Part model, mm, in its own coordinate system. Face numbers are marked on the shaded views. A direction names the side the tool comes from. Round coordinates to 2 decimals unless told otherwise and drop trailing zeros. Loops run counter-clockwise (first coordinate to the right, second up) from the corner with the lowest first, then second, coordinate; pieces in that order, holes last. Notation, with made-up numbers: (1, 24.25) - (7, 24.25) arc R29 ccw to (7, 55.25) - close; hole circle Ø11 at (85.25, 55.5). An arc over 180 degrees is marked (long way). Put each result on its own line as item: value.
from build123d import *

# Parameters (mm, degrees)
IZIM1_W                     = 15
IZIM1_H                     = 25
IZIM1_R                     = 2.5
Y_KSEKLIK_EKSTR_ZYON1_DEPTH = 2
IZIM2_W                     = 15
IZIM2_H                     = 2
Y_KSEKLIK_EKSTR_ZYON2_DEPTH = 23
IZIM3_R                     = 2.5
KES_EKSTR_ZYON1_DEPTH       = 13


with BuildPart() as part:
    # Çizim1 → Yükseklik-Ekstrüzyon1 (new body)
    with BuildSketch(Plane(origin=(0, 0, 0), x_dir=(1, 0, 0), z_dir=(0, 1, 0))):
        Rectangle(IZIM1_W, IZIM1_H)
        with Locations(Location((0, 8.75, 0), (0, 0, 270))):
            Circle(IZIM1_R, mode=Mode.SUBTRACT)
    extrude(amount=Y_KSEKLIK_EKSTR_ZYON1_DEPTH)

    # Çizim2 → Yükseklik-Ekstrüzyon2 (add)
    with BuildSketch(Plane(origin=(0, 2, 0), x_dir=(1, 0, 0), z_dir=(0, 1, 0))):
        with Locations((0, -11.5)):
            Rectangle(IZIM2_W, IZIM2_H)
    extrude(amount=Y_KSEKLIK_EKSTR_ZYON2_DEPTH)

    # Çizim3 → Kes-Ekstrüzyon1 (cut)
    with BuildSketch(Plane(origin=(0, 0, 10.5), x_dir=(-1, 0, 0), z_dir=(0, 0, -1))):
        with Locations((0, 21.25)):
            Circle(IZIM3_R)
    extrude(amount=-KES_EKSTR_ZYON1_DEPTH, mode=Mode.SUBTRACT)


solid = part.part
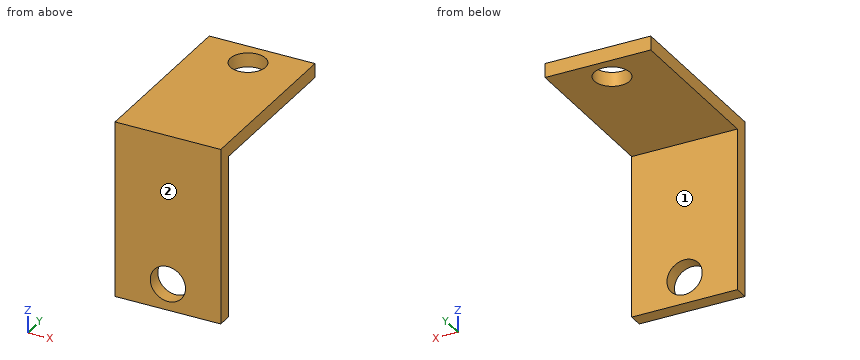
1. Band-saw the part on D-D (x = 4.25). List the corners of the cut face in (y, z).
A:
outline: (0, -12.5) - (2, -12.5) - (2, 10.5) - (25, 10.5) - (25, 12.5) - (0, 12.5) - close
2. Band-saw the part on B-B (y = 21.25). List the corners of the cut face in (x, z), plus the area to 3 significant figures.
A:
outline: (-7.5, 10.5) - (-2.5, 10.5) - (-2.5, 12.5) - (-7.5, 12.5) - close; (2.5, 10.5) - (7.5, 10.5) - (7.5, 12.5) - (2.5, 12.5) - close
area: 20.0 mm²
3. Pin check, flat tips, straight feed: P1, Ø7.5, axis at x = 2, y = 13, coming from the -Z side; P2, Ø6.5, axis at x = 0, z = -8.75, coming from the +Y side. Stop position of each tip, or through.
A:
P1: stops at z = 10.5
P2: stops at y = 2
4. Band-saw the part on C-C (x = 0). List the corners of the cut face in (y, z).
A:
outline: (0, -12.5) - (2, -12.5) - (2, -11.25) - (0, -11.25) - close; (0, -6.25) - (2, -6.25) - (2, 10.5) - (18.75, 10.5) - (18.75, 12.5) - (0, 12.5) - close; (23.75, 10.5) - (25, 10.5) - (25, 12.5) - (23.75, 12.5) - close
5. Band-saw the part on A-A (z = -8.75). List the corners of the cut face in (x, y), plus the area to 3 significant figures.
A:
outline: (-7.5, 0) - (-2.5, 0) - (-2.5, 2) - (-7.5, 2) - close; (2.5, 0) - (7.5, 0) - (7.5, 2) - (2.5, 2) - close
area: 20.0 mm²
6. Tool access for the marked faces 1 and 2: list every direction of +Z, -Z, +X, -X, +Y, -Y with a clear straight run to the whole face (end or side of a thin tool).
A:
face 1: -Z, +X, -X, +Y
face 2: +Z, -Z, +X, -X, -Y
7. Probe line 1 along Y through (x, z) = (0, 11.65); line 2 along X through (y, z) = (1.4, -8.75); line 3 along Z through (x, y) = (6.5, 14). List the from-to ranges inside material, lowest first. Write a range as [from, to].
A:
line 1: y = [0, 18.75], [23.75, 25]
line 2: x = [-7.5, -2.5], [2.5, 7.5]
line 3: z = [10.5, 12.5]
